Autodesk Inventor part; units mm, degrees
ref_plane "Work Plane1" through (29, 0, 0) normal (0, -1, 0) x (1, 0, 0)
ref_plane "YZ Plane" through (0, 0, 0) normal (1, 0, 0) x (0, 1, 0)
ref_plane "XZ Plane" through (0, 0, 0) normal (0, 1, 0) x (-1, 0, 0)
sketch "スケッチ1" plane through (0, 0, 0) normal (0, 0, 1) x (1, 0, 0)
  line L0 (-0.7333, 0) -> (8, 0)
  line L1 (8, 0) -> (8, 1.25)
  line L2 (8, 1.25) -> (1.35, 1.25)
  line L3 (1.35, 1.25) -> (1.0738, 1.25)
  line L4 (1.0738, 1.25) -> (0, 1.25)
  line L5 (0, 1.25) -> (0, 2.25)
  line L6 (0, 2.25) -> (-2.5, 2.25)
  line L7 (-2.5, 2.25) -> (-2.5, 1.1547)
  line L8 (-2.5, 1.1547) -> (-1.4, 1.1547)
  line L9 (-1.4, 1.1547) -> (-0.7333, 0)
  line L10 (-4.6, 0) -> (10.1, 0)
  line L11 (0, -0.45) -> (0, 2.7)
  line L12 (1.35, 1.25) -> (0, 1.25) construction
  dimension "d1" = 6.65
  dimension "d2" = 0.2762
  dimension "d3" = 2.5
  dimension "d4" = 1.1
  dimension "d5" = 60
  dimension "d6" = 2.5
  dimension "d7" = 2.5
  dimension "d8" = 2.3094
  dimension "d9" = 4.5
  dimension "d26" = 8
revolve "ボディ" add sketch "スケッチ1" angle 360 about axis through (-0.7333, 0, 0) along (1, 0, 0)
sketch "スケッチ2" plane through (-2.5, 0, 0) normal (-1, 0, 0) x (0, 0, 1)
  circle A0 centre (0, 0) radius 1.1547
  line L0 (0, -3.15) -> (0, 3.15)
  line L1 (-3.15, 0) -> (3.15, 0)
  line L2 (1.1547, 0) -> (0.5774, -1)
  line L3 (0.5774, -1) -> (-0.5774, -1)
  line L4 (-0.5774, -1) -> (-1.1547, 0)
  line L5 (-1.1547, 0) -> (-0.5774, 1)
  line L6 (-0.5774, 1) -> (0.5774, 1)
  line L7 (0.5774, 1) -> (1.1547, 0)
extrude "長穴" add sketch "スケッチ2" against normal up to next contours L7 A0 | A0 L2 | L6 L0 A0 | A0 L0 L3 | L0 L6 A0 | A0 L3 L0 | L4 A0 | A0 L5
fillet "フィレット1" radius 0.25 1 edges at (-2.5, -2.25, 0)
thread "ねじ"
chamfer "面取り1" distance 0.2761 distance2 0.2761 1 edges at (8, -1.25, 0) measured on face at (8, 0.4797, 0.7189)
ref_plane "Work Plane1" through (29, 0, 0) normal (0, -1, 0) x (1, 0, 0)
fillet "Fillet2" radius 0.1 1 edges at (0, -1.25, 0)
equation "\"d30\" = R"
equation "\"d17\" = RR"
equation "\"d13\" = GEL"
equation "\"d15\" = -0.5 * SPD + 0.5 * GD"
equation "\"d16\" = GUL"
equation "\"d1\" = GEL"
equation "\"d3\" = KOH"
equation "\"d4\" = INTI"
equation "\"d6\" = GD"
equation "\"d7\" = BDM"
equation "\"d8\" = 1.1547 * SW"
equation "\"d9\" = KOD"
equation "\"d26\" = NLG"
equation "\"GD\" = NND"
equation "\"NLG\" = 8"
equation "\"GEL\" = 6.65"
equation "\"KOD\" = 4.5"
equation "\"KOH\" = 2.5"
equation "\"INTI\" = 1.1"
equation "\"GAL\" = 0.61345 * PTC"
equation "\"GUL\" = 0.61345 * PTC"
equation "\"BDM\" = NND"
equation "\"SW\" = 2"
equation "\"RR\" = 0.25"
equation "\"SPD\" = NND - 1.2269 * PTC"
equation "\"R\" = 0.1"
equation "\"PHH\" = 0.1"
equation "\"GD1\" = THREADDIA - 1.2269 * PTC"
equation "\"THREADDIA\" = 2.5"
equation "\"FAWI\" = 45deg"
equation "\"PTC\" = 0.45"
equation "\"NND\" = 2.5"
equation "\"TOA\" = 30deg"
equation "\"E0\" = 1.155 * SW"
properties part number "JIS B 1176 - M2.5 x 8" material "鋼、軟鋼"
Input: part model. Units: mm. Frame: model coordinates. A direction names the side the tool comes from. Give positions to 0.01 mm unless a question says otherwise; leave off trailing zeros. Write each loop counter-clockwise with the first axis right and the second up, starting at its lowest first coordinate (ties: lowest second). Pieces come first, ordered by that corner, then holes. Notation, with made-up numbers: M 11,31.25 L 23,31.25 A31 cw 23,59.25 Z; hole C -27.75,2 d3. An arc over 180 degrees is marked long. Use one line per item in the form item = value.
1. Ray query, L1, parallel to X at y = 0.1, z = -1.6; L2, parallel to Z at x = -1, y = 0.25; L3, parallel to Z at x = 1, y = 0.5. Return the intervals inside material, ascending.
Outcome:
L1 = -2.5 to 0
L2 = -2.24 to -0.39, 0.39 to 2.24
L3 = -1.15 to 1.15
2. Mould query, pull axis Z, two halves, no side actions, for faces 4 (the face through (-0.775, 0.069, -0.022)), 5 (the face through (-1.14, -0.29, -2.23)), 6 (the face through (0, 0.5, -1.5)). Classes: released by +Z, released by -Z, zero draft, split by the parting line, or undercut.
Outcome:
face_4 = undercut
face_5 = split by the parting line
face_6 = zero draft
3. Cut plane B-B on x = -0.5. Return loops of the section in (y, z).
Outcome:
outline = C 0,0 d4.5
4. Cut plane A-A on x = 1. Return loops of the section in (y, z), and give its area (3 significant figures).
Outcome:
outline = C 0,0 d2.5
area = 4.91 mm²
5. First-contact query: P1, Ø1.5, axis at x = 3, y = -1.5, coming from the +Z side; P2, Ø1, axis at x = 2.5, z = -1, coming from the -Y side; P3, Ø1.5, axis at x = 2, z = 0, coming from the -Y side. Flat tips, straight axial feed; report the tip coordinate or a pass-through.
Outcome:
P1 = 1
P2 = -1.15
P3 = -1.25
6. Reachability of faces 1 (the face through (-1.91, 0.49, -0.87)), 2 (the face through (-2.5, -1, 1)), 3 (the face through (3.86, -0.27, 1.22)) from +Z, -Z, +X, -X, +Y, -Y: full face, straight path, thin tool, end or side. Return the list, or none.
Outcome:
face_1 = -X
face_2 = +Z, -Z, -X, +Y, -Y
face_3 = +X
